Here's how the part is built. I have some questions about the finished solid (model axes, mm). Face numbers are marked on the shaded views. A direction names the side the tool comes from. Give positions to 0.01 mm unless a question says otherwise; leave off trailing zeros. Write each loop counter-clockwise with the first axis right and the second up, starting at its lowest first coordinate (ties: lowest second). Pieces come first, ordered by that corner, then holes. Notation, with made-up numbers: (30, 33.5) - (59, 33.5) arc R29 cw to (59, 55.5) - close; hole circle Ø7 at (59.25, -38.5). An arc over 180 degrees is marked (long way). One line per item, written item: value. Start each with the question number.
1) Imagine slicing it at C-C on y = 16.25. Write out the boundary of the cut face in (x, z) (3 decimals), plus the area to 3 significant figures.
2) Imagine slicing it at B-B on x = 0. Write out the boundary of the cut face in (y, z) (3 decimals), plus the area to 3 significant figures.
3) Imagine slicing it at A-A on z = 0. Write out the boundary of the cut face in (x, y) (3 decimals).
4) I'm going to push flat-ended pins straight in: P1, Ø1.5, axis at y = 23, z = 0, coming from the -X side (3 decimals); P2, Ø0.7, axis at x = -1.5, z = -0.5, coming from the +Y side; P3, Ø1.5, axis at y = 23, z = -0.5, coming from the +X side (3 decimals). Where does each tip first touch, or does it pass through?
5) On a 3-axis mill with a long thin cutter (end or side, diameter ignored), from which of +Z, -Z, +X, -X, +Y, -Y can I reach the whole of each face in a straight line? I mean the marked faces 1, 2 and 3. Say none if no direction works.
6) Imagine slicing it at D-D on x = 1.5. Write out the boundary of the cut face in (y, z), plus the area to 3 significant figures.
7) We'd pull the mould along X, two halves only. Please class the marked faces 4, 5, 6 and 7: +X half, -X half, draft (parallel to the pull), parting line (faces both ways), or undercut.
8) Please list where these lines run through material, in increasing order: L1, parallel to X at y = 0.65, z = 0 (3 decimals); L2, parallel to Y at x = -2.5, z = -1.25; L3, parallel to X at y = 21, z = 0 (3 decimals). Write a range as [from, to].
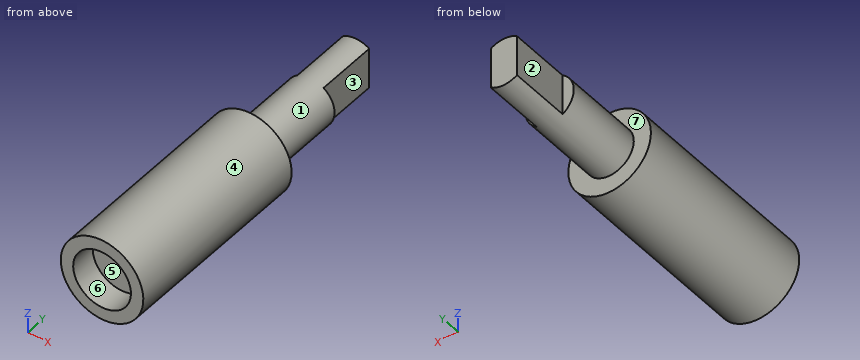
from build123d import *

# Parameters (mm, degrees)
SKETCH1_R           = 3.075
BOSS_EXTRUDE1_DEPTH = 14.77
SKETCH2_R           = 1.8
BOSS_EXTRUDE2_DEPTH = 5.98
BOSS_EXTRUDE3_DEPTH = 4.55
SKETCH4_R           = 2.15
CUT_EXTRUDE1_DEPTH  = 1.95


with BuildPart() as part:
    # Sketch1 → Boss-Extrude1 (new body)
    with BuildSketch(Plane(origin=(0, 0, 0), x_dir=(1, 0, 0), z_dir=(0, 1, 0))):
        with Locations(Location((0, 0, 0), (0, 0, 270))):
            Circle(SKETCH1_R)
    extrude(amount=BOSS_EXTRUDE1_DEPTH)

    # Sketch2 → Boss-Extrude2 (add)
    with BuildSketch(Plane(origin=(0, 14.77, 0), x_dir=(1, 0, 0), z_dir=(0, 1, 0))):
        with Locations(Location((0, 0, 0), (0, 0, 90))):
            Circle(SKETCH2_R)
    extrude(amount=BOSS_EXTRUDE2_DEPTH)

    # Sketch3 → Boss-Extrude3 (add)
    with BuildSketch(Plane(origin=(0, 20.75, 0), x_dir=(1, 0, 0), z_dir=(0, 1, 0))):
        with BuildLine():
            Line((-0.975, 1.513068075), (-0.975, -1.513068075))
            ThreePointArc((-0.975, -1.513068075), (0, -1.8), (0.975, -1.513068075))
            Line((0.975, -1.513068075), (0.975, 1.513068075))
            ThreePointArc((0.975, 1.513068075), (0, 1.8), (-0.975, 1.513068075))
        make_face()
    extrude(amount=BOSS_EXTRUDE3_DEPTH)

    # Sketch4 → Cut-Extrude1 (cut)
    with BuildSketch(Plane.XZ):
        with Locations(Location((0, 0, 0), (0, 0, 270))):
            Circle(SKETCH4_R)
    extrude(amount=-CUT_EXTRUDE1_DEPTH, mode=Mode.SUBTRACT)


solid = part.part
Numbers:
1. outline: circle Ø3.6 at (0, 0)
1. area: 10.2 mm^2
2. outline: (0, -3.075) - (14.77, -3.075) - (14.77, -1.8) - (25.3, -1.8) - (25.3, 1.8) - (14.77, 1.8) - (14.77, 3.075) - (0, 3.075) - (0, 2.15) - (1.95, 2.15) - (1.95, -2.15) - (0, -2.15) - close
2. area: 120 mm^2
3. outline: (-3.075, 0) - (-2.15, 0) - (-2.15, 1.95) - (2.15, 1.95) - (2.15, 0) - (3.075, 0) - (3.075, 14.77) - (1.8, 14.77) - (1.8, 20.75) - (0.975, 20.75) - (0.975, 25.3) - (-0.975, 25.3) - (-0.975, 20.75) - (-1.8, 20.75) - (-1.8, 14.77) - (-3.075, 14.77) - close
4. P1: x = -0.975
4. P2: y = 20.75
4. P3: x = 0.975
5. face 1: +Y
5. face 2: +Z, -Z, -X, +Y
5. face 3: +Z, -Z, +X, +Y
6. outline: (0, -2.68) - (14.77, -2.68) - (14.77, -0.99) - (20.75, -0.99) - (20.75, 0.99) - (14.77, 0.99) - (14.77, 2.68) - (0, 2.68) - (0, 1.54) - (1.95, 1.54) - (1.95, -1.54) - (0, -1.54) - close
6. area: 85.2 mm^2
7. face 4: parting line
7. face 5: undercut
7. face 6: undercut
7. face 7: draft
8. L1: [-3.075, -2.15], [2.15, 3.075]
8. L2: [0, 14.77]
8. L3: [-0.975, 0.975]
